```python
from build123d import *

# Parameters (mm, degrees)
SKETCH1_R           = 2.032
BOSS_EXTRUDE1_DEPTH = 3.175
FILLET1_R           = 6.35
FILLET2_R           = 3.175


with BuildPart() as part:
    # Sketch1 → Boss-Extrude1 (new body)
    with BuildSketch(Plane(origin=(0, 0, 0), x_dir=(1, 0, 0), z_dir=(0, 1, 0))):
        Polygon((44.45, 9.525), (45.451117841, 0), (72.438617841, 0), (71.4375, 9.525), (64.29375, 60.325), (51.59375, 60.325), align=None)
        with Locations(Location((50.8, 4.7625, 0), (0, 0, 270))):
            Circle(SKETCH1_R, mode=Mode.SUBTRACT)
        with Locations(Location((63.5, 4.7625, 0), (0, 0, 270))):
            Circle(SKETCH1_R, mode=Mode.SUBTRACT)
    extrude(amount=BOSS_EXTRUDE1_DEPTH)

    # Fillet1
    fillet1_edges = [part.edges().sort_by_distance(p)[0] for p in [
        (51.59375, 1.5875, -60.325),
        (64.29375, 1.5875, -60.325),
    ]]
    fillet(fillet1_edges, radius=FILLET1_R)

    # Fillet2
    fillet2_edges = [part.edges().sort_by_distance(p)[0] for p in [
        (72.438617841, 1.5875, 0),
        (45.451117841, 1.5875, 0),
    ]]
    fillet(fillet2_edges, radius=FILLET2_R)


solid = part.part
```
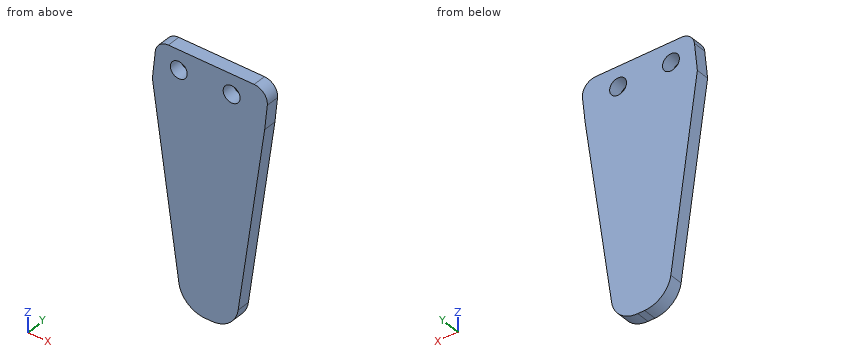
Input: part model. Units: mm. Frame: model coordinates. Give positions to 0.01 mm unless a question says otherwise; leave off trailing zeros. Order: outer loops, then holes, each group sorted by start corner. A loop starts at its lowest first (then second) coordinate and runs counter-clockwise, first axis right, second up. Notation, with made-up numbers: (41.5, -10) - (80.5, -10) arc R12 ccw to (80.5, -2) - close; hole circle Ø10 at (10, 14.25). An arc over 180 degrees is marked (long way). Use a Markdown table: item, result.
(1) Line query: line 1 (X direction, y = 1.45, z = -5.5); line 2 (X direction, y = 2.6, z = -5); line 3 (X direction, y = 0.65, z = -39.5). Output: solid intervals per line, ascending. Write a range as from..to.
Computed values:
| item | result |
|---|---|
| line 1 | x = 44.87..48.91, 52.69..61.61, 65.39..71.86 |
| line 2 | x = 44.93..48.78, 52.82..61.48, 65.52..71.91 |
| line 3 | x = 48.67..67.22 |
(2) Section query D-D (x = 67.5). Output: boundary loops of the cut face in (y, z) (3 decimals).
Computed values:
| item | result |
|---|---|
| outline | (0, -37.525) - (3.175, -37.525) - (3.175, 0) - (0, 0) - close |
(3) Section query A-A (y = 1.2). State how many separate pieces and enclosed holes the cut face has, then the cut area to 3 significant figures.
Computed values:
| item | result |
|---|---|
| separate pieces | 1 |
| enclosed holes | 2 |
| area | 1,220 mm2 |
(4) Section query B-B (x = 63.5). Output: boundary loops of the cut face in (y, z) (1 decimal).
Computed values:
| item | result |
|---|---|
| outline | (0, -58.2) - (3.2, -58.2) - (3.2, -6.8) - (0, -6.8) - close; (0, -2.7) - (3.2, -2.7) - (3.2, 0) - (0, 0) - close |
(5) Section query C-C (z = -19). Output: boundary loops of the cut face in (x, y) (3 decimals).
Computed values:
| item | result |
|---|---|
| outline | (45.782, 0) - (70.105, 0) - (70.105, 3.175) - (45.782, 3.175) - close |
(6) Pin query (flat end, axial travel): pin 1 (1 mm diameter, centred on x = 56, y = 2.5, fed in from -Z); pin 2 (3.5 mm diameter, centred on x = 50.8, z = -4.76, fed in from +Y); pin 3 (4.5 mm diameter, centred on x = 63.5, z = -4.76, fed in from -Y). Return the tip coordinate at first contact, or that it passes through.
Computed values:
| item | result |
|---|---|
| pin 1 | stops at z = -60.3 |
| pin 2 | passes through |
| pin 3 | stops at y = 0 |
